Could you check a few things on this model? Use its own coordinates, in mm. A direction names the side the tool comes from. Round coordinates to 2 decimals unless told otherwise and drop trailing zeros. Loops run counter-clockwise (first coordinate to the right, second up) from the corner with the lowest first, then second, coordinate; pieces in that order, holes last.
Autodesk Inventor part; units mm, degrees
ref_plane "Počáteční rovina" through (0, 0, 0) normal (0, 0, 1) x (1, 0, 0)
ref_plane "Koncová rovina" through (0, 0, 1075) normal (0, 0, 1) x (1, 0, 0)
ref_plane "Pracovní rovina4" through (517.5027, -11.5, 534.9973) normal (0, 0, 1) x (0, -1, 0)
ref_plane "Počáteční rovina" through (0, 0, 0) normal (0, 0, 1) x (1, 0, 0)
ref_plane "Koncová rovina" through (0, 0, 1075) normal (0, 0, 1) x (1, 0, 0)
sketch "Náčrt1" plane through (0, 0, 0) normal (0, 0, 1) x (1, 0, 0)
  line L0 (-11.5, 17.5) -> (11.5, 17.5)
  line L1 (17.5, 11.5) -> (17.5, -11.5)
  line L2 (11.5, -17.5) -> (-11.5, -17.5)
  line L3 (-17.5, -11.5) -> (-17.5, 11.5)
  arc A0 (-11.5, 17.5) -> (-17.5, 11.5) centre (-11.5, 11.5) ccw
  arc A1 (17.5, 11.5) -> (11.5, 17.5) centre (11.5, 11.5) ccw
  arc A2 (11.5, -17.5) -> (17.5, -11.5) centre (11.5, -11.5) ccw
  arc A3 (-17.5, -11.5) -> (-11.5, -17.5) centre (-11.5, -11.5) ccw
  line L4 (-26.2397, 0) -> (26.2397, 0) construction
  line L5 (0, -26.2397) -> (0, 26.2397) construction
  arc A4 (-11.5, 14.5) -> (-14.5, 11.5) centre (-11.5, 11.5) ccw
  line L6 (-11.5, 14.5) -> (11.5, 14.5)
  arc A5 (14.5, 11.5) -> (11.5, 14.5) centre (11.5, 11.5) ccw
  line L7 (14.5, 11.5) -> (14.5, -11.5)
  arc A6 (11.5, -14.5) -> (14.5, -11.5) centre (11.5, -11.5) ccw
  line L8 (11.5, -14.5) -> (-11.5, -14.5)
  arc A7 (-14.5, -11.5) -> (-11.5, -14.5) centre (-11.5, -11.5) ccw
  line L9 (-14.5, -11.5) -> (-14.5, 11.5)
  point P0 (-17.5, 17.5)
  point P1 (17.5, -17.5)
  point P2 (17.5, 17.5)
  dimension "b" = 35
  dimension "msp_r" = 6
  dimension "d8" = 17.5
  dimension "d9" = 17.5
  dimension "d10" = 3
extrude "Těleso" add sketch "Náčrt1" along normal blind 1070
sketch "Sketch2" plane through (0, 0, 0) normal (0, 0, 1) x (1, 0, 0)
  line L0 (0, 0) -> (10, 0)
ref_plane "Work Plane3" through (0, 0, 0) normal (0, -1, 0) x (1, 0, 0)
sketch "Sketch3" plane through (0, 0, 0) normal (0, -1, 0) x (1, 0, 0)
  line L0 (-2, 0) -> (12, 0)
  line L1 (-2, 1075) -> (12, 1075)
  dimension "d14" = 1075
sketch "Náčrt4" plane through (11.5, 17.5, 1075) normal (0, 1, 0) x (1, 0, 0)
  line L0 (-23, 1075) -> (-29, 1075)
  line L1 (6, 1075) -> (6, 5) construction
  line L2 (-29, 1075) -> (6, 1075)
  line L3 (6, 1075) -> (6, 1040.0004)
  line L4 (-29, 1075) -> (6, 1040.0004)
  line L5 (-29, 1075) -> (-29, 5) construction
  line L6 (-23, 5) -> (-29, 5)
  line L7 (6, 5) -> (-29, 5)
  line L8 (-29, 5) -> (6, 40)
  line L9 (6, 40) -> (6, 5)
  point P0 (-11.5, 1075)
  dimension "d15" = 45
  dimension "d19" = 45
extrude "Vysunutí2" cut sketch "Náčrt4" against normal through all
ref_plane "Pracovní rovina4" through (517.5027, -11.5, 534.9973) normal (0, 0, 1) x (0, -1, 0)
equation "\"msp_r\" = 2 * ParT"
equation "\"d8\" = d9"
equation "\"d9\" = 0.5 * b"
equation "\"d10\" = ParT"
equation "\"G_OFFSET_START\" = 0"
equation "\"G_OFFSET_END\" = 0"
equation "\"d12\" = G_OFFSET_END + B_L"
equation "\"G_L\" = d14"
equation "\"B_L\" = 1075"
properties part number "DD_KVD_003_03" material "Nerezová ocel"
Item 1: If we section it at C-C, the plane z = 763.5: Please give me the cut outline in (x, y), then the cut area to 3 significant figures.
Results list:
outline: (-17.5, -11.5) arc R6 ccw to (-11.5, -17.5) - (11.5, -17.5) arc R6 ccw to (17.5, -11.5) - (17.5, 11.5) arc R6 ccw to (11.5, 17.5) - (-11.5, 17.5) arc R6 ccw to (-17.5, 11.5) - close; hole (-14.5, -11.5) arc R3 ccw to (-11.5, -14.5) - (11.5, -14.5) arc R3 ccw to (14.5, -11.5) - (14.5, 11.5) arc R3 ccw to (11.5, 14.5) - (-11.5, 14.5) arc R3 ccw to (-14.5, 11.5) - close
area: 361 mm2
Item 2: Will these pins go through, and if not, where does the flat tip stop? pin 1 (2 mm diameter, centred on x = -13.5, z = 786.5, fed in from -Y); pin 2 (10 mm diameter, centred on x = -13.5, y = -7, fed in from -Z).
Results list:
pin 1: stops at y = -17.42
pin 2: stops at z = 0
Item 3: If we section it at A-A, the plane y = 1.5: Please give me the cut outline in (x, z), then the cut area to 3 significant figures.
Results list:
outline: (-17.5, 0) - (-14.5, 3) - (-14.5, 1067) - (-17.5, 1070) - close; (14.5, 32) - (17.5, 35) - (17.5, 1035) - (14.5, 1038) - close
area: 6,210 mm2
Item 4: If we section it at B-B, the plane x = 4: Please give me the cut outline in (y, z).
Results list:
outline: (-17.5, 21.5) - (-14.5, 21.5) - (-14.5, 1048.5) - (-17.5, 1048.5) - close; (14.5, 21.5) - (17.5, 21.5) - (17.5, 1048.5) - (14.5, 1048.5) - close
Item 5: We'd pull the mould along X, two halves only. Please class faces 1 (the flat face through (0, 17.5, 528)), 2 (the flat face through (0, 14.5, 528)), 3 (the flat face through (-17.5, 0, 528)): released by +X, released by -X, zero draft, split by the parting line, or undercut.
Results list:
face 1: zero draft
face 2: undercut
face 3: released by -X
Item 6: For faces 4 (the flat face through (0, -14.5, 528)), 5 (the flat face through (-0.2, -15.3, 1052.7)), which set-ups out of +Z, -Z, +X, -X, +Y, -Y let a thin tool reach every point of the face, with its end or its side?
Results list:
face 4: +Z, -Z
face 5: +Z, +X, +Y, -Y
Item 7: If I drill on line 1 along Y through (x, z) = (-0.5, 479); line 2 along X through (y, z) = (-12.5, 616), over which ranges is the centre line in solid material (lowest first)?
Results list:
line 1: y = -17.5 to -14.5, 14.5 to 17.5
line 2: x = -17.42 to -14.33, 14.33 to 17.42
